```python
from build123d import *

# Parameters (mm, degrees)
SKETCH_1_R                   = 33.5
SKETCH_1_R_2                 = 11.5
SKETCH_1_W                   = 80
SKETCH_1_H                   = 20
SKETCH_1_R_3                 = 2.1
EXTRUDE_1_DEPTH              = 6
SKETCH_3_W                   = 80
SKETCH_3_H                   = 3
EXTRUDE_2_DEPTH              = 6
FILLET_1_R                   = 5
EXTRUDE_START                = -6
EXTRUDE_3_DEPTH              = 6
SKETCH_5_R                   = 2
CUT_EXTRUDE_1_DEPTH          = 126.686116974
HOLE_WIZARD_M4_1_D           = 4.3
HOLE_WIZARD_M4_1_DEPTH       = 10
HOLE_WIZARD_M4_1_CSINK_D     = 8.96
HOLE_WIZARD_M4_1_CSINK_ANGLE = 90
HOLE_WIZARD_M4_1_TIP         = 1.291850331
SKETCH_8_R                   = 2.1
CUT_EXTRUDE_2_DEPTH          = 10
HOLE_WIZARD_M4_2_D           = 4.3
HOLE_WIZARD_M4_2_DEPTH       = 10
HOLE_WIZARD_M4_2_CSINK_D     = 8.96
HOLE_WIZARD_M4_2_CSINK_ANGLE = 90
HOLE_WIZARD_M4_2_TIP         = 1.291850331
CHAMFER_1_SIZE               = 5
CUT_EXTRUDE_3_DEPTH          = 126.686116974
SKETCH_13_W                  = 50
SKETCH_13_H                  = 20
CUT_EXTRUDE_5_DEPTH          = 10
FILLET_3_R                   = 3
FILLET_4_R                   = 6
FILLET_5_R                   = 5
FILLET_6_R                   = 1.5
FILLET_7_R                   = 5


with BuildPart() as part:
    # 草图1 → 凸台-拉伸1 (new body)
    # profile 1 of 3: a face of its own
    with BuildSketch(Plane.XY):
        with Locations((0, 85.5)):
            Circle(SKETCH_1_R)
        with Locations((0, 85.5)):
            Circle(SKETCH_1_R_2, mode=Mode.SUBTRACT)
    # profile 2 of 3: a face of its own
    with BuildSketch(Plane.XY):
        with BuildLine():
            Line((-33.38100662, 88.32106311), (-40, 10))
            Line((-40, 10), (40, 10))
            Line((40, 10), (33.38100662, 88.32106311))
            ThreePointArc((33.38100662, 88.32106311), (33.470238435, 86.911785792), (33.5, 85.5))
            ThreePointArc((33.5, 85.5), (-1.411785792, 52.029761565), (-33.38100662, 88.32106311))
        make_face()
    # profile 3 of 3: a face of its own
    with BuildSketch(Plane.XY):
        Rectangle(SKETCH_1_W, SKETCH_1_H)
        with Locations((-30, 7.5)):
            Circle(SKETCH_1_R_3, mode=Mode.SUBTRACT)
        with Locations((30, 7.5)):
            Circle(SKETCH_1_R_3, mode=Mode.SUBTRACT)
        with Locations((30, -7.5)):
            Circle(SKETCH_1_R_3, mode=Mode.SUBTRACT)
        with Locations((-30, -7.5)):
            Circle(SKETCH_1_R_3, mode=Mode.SUBTRACT)
    extrude(amount=EXTRUDE_1_DEPTH)

    # 草图3 → 凸台-拉伸2 (add)
    with BuildSketch(Plane.XY.offset(6)):
        with Locations((0, -11.5)):
            Rectangle(SKETCH_3_W, SKETCH_3_H)
    extrude(amount=-EXTRUDE_2_DEPTH)

    # 圆角1
    fillet_1_edges = [part.edges().sort_by_distance(p)[0] for p in [
        (-40, -13, 3),
        (40, -13, 3),
    ]]
    fillet(fillet_1_edges, radius=FILLET_1_R)

    # 草图4 → 凸台-拉伸3 (add)
    with BuildSketch(Plane.XY.offset(6).offset(EXTRUDE_START)):
        with BuildLine():
            Line((33.38100662, 88.32106311), (11.148614395, 88.32106311))
            ThreePointArc((11.148614395, 88.32106311), (-1.418941021, 96.91212541), (-11.499998905, 85.50501918))
            Line((-11.499998905, 85.50501918), (-33.61899338, 85.50501918))
            Line((-33.61899338, 85.50501918), (-33.61899338, 119))
            Line((-33.61899338, 119), (33.38100662, 119))
            Line((33.38100662, 119), (33.38100662, 88.32106311))
        make_face()
    extrude(amount=EXTRUDE_3_DEPTH)

    # 草图5 → 切除-拉伸1 (cut, through all)
    with BuildSketch(Plane.XY.offset(6)):
        with Locations((-17.901394117, 83.618487661)):
            Circle(SKETCH_5_R)
        with Locations((17.386664873, 90.158742812)):
            Circle(SKETCH_5_R)
    extrude(amount=-CUT_EXTRUDE_1_DEPTH, mode=Mode.SUBTRACT)

    # M4 六角凹锥坑螺钉的锥形沉头孔1
    with Locations(Plane(origin=(0, 0, 0), x_dir=(-1, 0, 0), z_dir=(0, 0, -1))):
        with Locations((-17.386664873, 90.158742812), (17.901394117, 83.618487661)):
            CounterSinkHole(HOLE_WIZARD_M4_1_D / 2, HOLE_WIZARD_M4_1_CSINK_D / 2, depth=HOLE_WIZARD_M4_1_DEPTH, counter_sink_angle=HOLE_WIZARD_M4_1_CSINK_ANGLE)
            with Locations((0, 0, -(HOLE_WIZARD_M4_1_DEPTH + HOLE_WIZARD_M4_1_TIP / 2))):  # 118° drill point
                Cone(0, HOLE_WIZARD_M4_1_D / 2, HOLE_WIZARD_M4_1_TIP, mode=Mode.SUBTRACT)

    # 草图8 → 切除-拉伸2 (cut)
    with BuildSketch(Plane.XY.offset(6)):
        with Locations((-12.118993381, 114)):
            Circle(SKETCH_8_R)
        with Locations((22.881006619, 114)):
            Circle(SKETCH_8_R)
    extrude(amount=-CUT_EXTRUDE_2_DEPTH, mode=Mode.SUBTRACT)

    # M4 六角凹锥坑螺钉的锥形沉头孔2
    with Locations(Plane(origin=(0, 0, 0), x_dir=(-1, 0, 0), z_dir=(0, 0, -1))):
        with Locations((-22.881006619, 114), (12.118993381, 114)):
            CounterSinkHole(HOLE_WIZARD_M4_2_D / 2, HOLE_WIZARD_M4_2_CSINK_D / 2, depth=HOLE_WIZARD_M4_2_DEPTH, counter_sink_angle=HOLE_WIZARD_M4_2_CSINK_ANGLE)
            with Locations((0, 0, -(HOLE_WIZARD_M4_2_DEPTH + HOLE_WIZARD_M4_2_TIP / 2))):  # 118° drill point
                Cone(0, HOLE_WIZARD_M4_2_D / 2, HOLE_WIZARD_M4_2_TIP, mode=Mode.SUBTRACT)

    # 倒角1
    chamfer_1_edges = [part.edges().sort_by_distance(p)[0] for p in [
        (33.38100662, 119, 3),
    ]]
    chamfer(chamfer_1_edges, length=CHAMFER_1_SIZE)

    # 草图11 → 切除-拉伸3 (cut, through all)
    with BuildSketch(Plane.XY.offset(6)):
        Polygon((-33.61899338, 119), (-16.422785999, 119), (-33.61899338, 85.50501918), align=None)
    extrude(amount=-CUT_EXTRUDE_3_DEPTH, mode=Mode.SUBTRACT)

    # 草图13 → 切除-拉伸5 (cut)
    with BuildSketch(Plane.XY.offset(6)):
        with BuildLine():
            Line((-29.15457937, 67.081692819), (-19.750016495, 29.647135893))
            Line((-19.750016495, 29.647135893), (-3.346711376, 58.058493772))
            ThreePointArc((-3.346711376, 58.058493772), (-20.530627933, 66.987030012), (-27.640305628, 84.999754146))
            Line((-27.640305628, 84.999754146), (-29.15457937, 67.081692819))
        make_face()
        Polygon((-24.106901542, 22.100789629), (-30.830808938, 47.247244556), (-33.302523575, 18), (-23.010391923, 18), align=None)
        Polygon((-3, 46.65901549), (-17.649366774, 21.285567939), (-19.546290308, 18), (-3, 18), align=None)
        with BuildLine():
            Line((29.15457937, 67.081692819), (27.640305628, 84.999754146))
            ThreePointArc((27.640305628, 84.999754146), (20.530627933, 66.987030012), (3.346711376, 58.058493772))
            Line((3.346711376, 58.058493772), (19.750016495, 29.647135893))
            Line((19.750016495, 29.647135893), (29.15457937, 67.081692819))
        make_face()
        Polygon((17.649366774, 21.285567939), (3, 46.65901549), (3, 18), (19.546290308, 18), align=None)
        Polygon((33.302523575, 18), (30.711815557, 48.65526652), (24.060716784, 22.180783977), (23.010391923, 18), align=None)
        with Locations((0, 2)):
            Rectangle(SKETCH_13_W, SKETCH_13_H)
    extrude(amount=-CUT_EXTRUDE_5_DEPTH, mode=Mode.SUBTRACT)

    # 圆角3
    fillet_3_edges = [part.edges().sort_by_distance(p)[0] for p in [
        (25, -8, 3),
        (-25, -8, 3),
        (-25, 12, 3),
        (25, 12, 3),
    ]]
    fillet(fillet_3_edges, radius=FILLET_3_R)

    # 圆角4
    # the kernel refuses this fillet: 6 mm, written as the material it adds along each edge
    with BuildSketch(Plane(origin=(27.640305628, 84.999754146, 6), x_dir=(0.08421083909463391, -0.996447958791114, 0), z_dir=(0, 0, -1))) as fillet_4_piece_1:
        with BuildLine():
            CenterArc((21.827755911, 4.605393907), FILLET_4_R, 137.118904636, 93.016882278)
            Line((17.431151142, 8.688268692), (17.343219046, 8.769926188))
            ThreePointArc((17.343219046, 8.769926188), (9.452514246, 2.865624658), (-0.012267388, 0.119371316))
            Line((-0.012267388, 0.119371316), (0, -0.12))
            ThreePointArc((0, -0.12), (8.990966949, -0.12), (17.905017457, -0.092107878))
            Line((17.905017457, -0.092107878), (17.981933897, 0))
        make_face()
    extrude(amount=6)
    with BuildSketch(Plane(origin=(-27.640305628, 84.999754146, 6), x_dir=(-0.08421083909464076, -0.9964479587911135, 0), z_dir=(0, 0, -1))) as fillet_4_piece_2:
        with BuildLine():
            CenterArc((21.827755911, -4.605393907), FILLET_4_R, 129.864213086, 93.016882278)
            Line((17.431151142, -8.688268692), (17.343219046, -8.769926188))
            ThreePointArc((17.343219046, -8.769926188), (9.452514246, -2.865624658), (-0.012267388, -0.119371316))
            Line((-0.012267388, -0.119371316), (0, 0.12))
            ThreePointArc((0, 0.12), (8.990966949, 0.12), (17.905017457, 0.092107878))
            Line((17.905017457, 0.092107878), (17.981933897, 0))
        make_face()
    extrude(amount=6)

    # 圆角5
    fillet_5_edges = [part.edges().sort_by_distance(p)[0] for p in [
        (3.346711376, 58.058493772, 3),
        (-3.346711376, 58.058493772, 3),
    ]]
    fillet(fillet_5_edges, radius=FILLET_5_R)

    # 圆角6
    fillet_6_edges = [part.edges().sort_by_distance(p)[0] for p in [
        (19.546290308, 18, 3),
        (3, 18, 3),
        (3, 46.65901549, 3),
        (19.750016495, 29.647135893, 3),
        (-19.546290308, 18, 3),
        (-3, 46.65901549, 3),
        (-3, 18, 3),
        (-23.010391923, 18, 3),
        (-33.302523575, 18, 3),
        (-30.830808938, 47.247244556, 3),
        (23.010391923, 18, 3),
        (30.711815557, 48.65526652, 3),
        (33.302523575, 18, 3),
        (-19.750016495, 29.647135893, 3),
    ]]
    fillet(fillet_6_edges, radius=FILLET_6_R)

    # 圆角7
    # the kernel refuses this fillet: 5 mm, written as the material it adds along each edge
    with BuildSketch(Plane(origin=(29.15457937, 67.081692819, 6), x_dir=(-0.2436552741241345, -0.9698619011959861, 0), z_dir=(0, 0, -1))) as fillet_7_piece_1:
        with BuildLine():
            CenterArc((6.41210713, 5), FILLET_7_R, 121.736562988, 148.263437012)
            Line((3.782034708, 9.252378047), (3.519027465, 9.677615851))
            ThreePointArc((3.519027465, 9.677615851), (2.06186763, 8.837638689), (-0.427669644, -0.25903412))
            Line((-0.427669644, -0.25903412), (0, -0.5))
            Line((0, -0.5), (6.41210713, -0.5))
            Line((6.41210713, -0.5), (6.41210713, 0))
        make_face()
    extrude(amount=6)
    with BuildSketch(Plane(origin=(-29.15457937, 67.081692819, 6), x_dir=(0.24365527412411786, -0.9698619011959904, 0), z_dir=(0, 0, -1))) as fillet_7_piece_2:
        with BuildLine():
            CenterArc((6.41210713, -5), FILLET_7_R, 90, 148.263437012)
            Line((3.782034708, -9.252378047), (3.519027465, -9.677615851))
            ThreePointArc((3.519027465, -9.677615851), (2.06186763, -8.837638689), (-0.427669644, 0.25903412))
            Line((-0.427669644, 0.25903412), (0, 0.5))
            Line((0, 0.5), (6.41210713, 0.5))
            Line((6.41210713, 0.5), (6.41210713, 0))
        make_face()
    extrude(amount=6)


solid = part.part
```
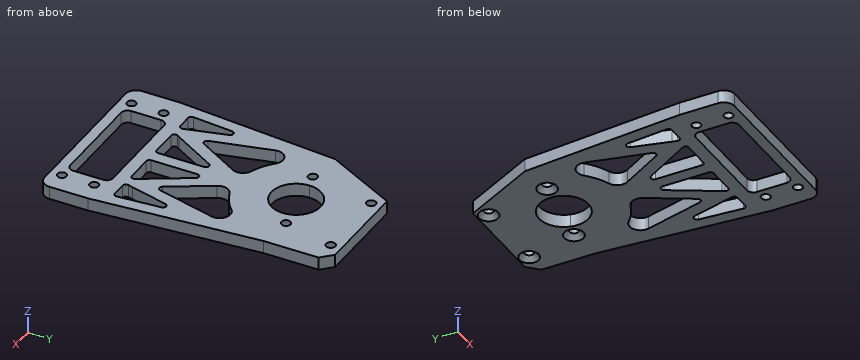
Work out the finished part from the listing and answer in its coordinate system (mm). Round coordinates to 2 decimals unless told otherwise and drop trailing zeros. Write each loop counter-clockwise with the first axis right and the second up, starting at its lowest first coordinate (ties: lowest second). Pieces come first, ordered by that corner, then holes.
1) Consider probe 1 along X at (y, z) = (60.5, 5.75); probe 2 along X at (y, z) = (85.5, 4.65); probe 3 along X at (y, z) = (4.5, 4). Determine where each line is inside the solid, lowest interval first.
2) A cutting plane is placed at B-B on x = 0. Determine the outline of the cut face in (y, z), and give its area (3 significant figures).
3) A cutting plane is placed at C-C on x = -30. Determine the outline of the cut face in (y, z).
4) Flat-ended cylindrical pins translate along their axes: P1, Ø6.5, axis at x = -30, y = -7.5, coming from the +Z side; P2, Ø3, axis at y = 27, z = 2.5, coming from the +X side; P3, Ø4, axis at x = 17.39, y = 90.16, coming from the -Z side; P4, Ø3, axis at y = 42.5, z = 1, coming from the +X side. Find the tip coordinate at first contact, or state that the pin passes through.
5) A cutting plane is placed at D-D on z = 1. Give the number of separate pieces and of enclosed holes in the cut face, and give its area (3 significant figures).
6) A cutting plane is placed at A-A on y = 7.5. Determine the outline of the cut face in (x, z).
Entries:
1. probe 1: x = -35.73 to -27.5, -11.8 to 11.8, 27.5 to 35.73
1. probe 2: x = -33.62 to -18.94, -16.86 to -11.5, 11.5 to 33.62
1. probe 3: x = -40 to -25, 25 to 40
2. outline: (-13, 0) - (-8, 0) - (-8, 6) - (-13, 6) - close; (12, 0) - (74, 0) - (74, 6) - (12, 6) - close; (97, 0) - (119, 0) - (119, 6) - (97, 6) - close
2. area: 534 mm2
3. outline: (-13, 0) - (-9.6, 0) - (-9.6, 6) - (-13, 6) - close; (-5.4, 0) - (5.4, 0) - (5.4, 6) - (-5.4, 6) - close; (9.6, 0) - (18, 0) - (18, 6) - (9.6, 6) - close; (40.06, 0) - (92.55, 0) - (92.55, 6) - (40.06, 6) - close
4. P1: stops at z = 6
4. P2: stops at x = 38.69
4. P3: passes through
4. P4: stops at x = 37.38
5. separate pieces: 1
5. enclosed holes: 16
5. area: 6,100 mm2
6. outline: (-40, 0) - (-32.1, 0) - (-32.1, 6) - (-40, 6) - close; (-27.9, 0) - (-25, 0) - (-25, 6) - (-27.9, 6) - close; (25, 0) - (27.9, 0) - (27.9, 6) - (25, 6) - close; (32.1, 0) - (40, 0) - (40, 6) - (32.1, 6) - close
